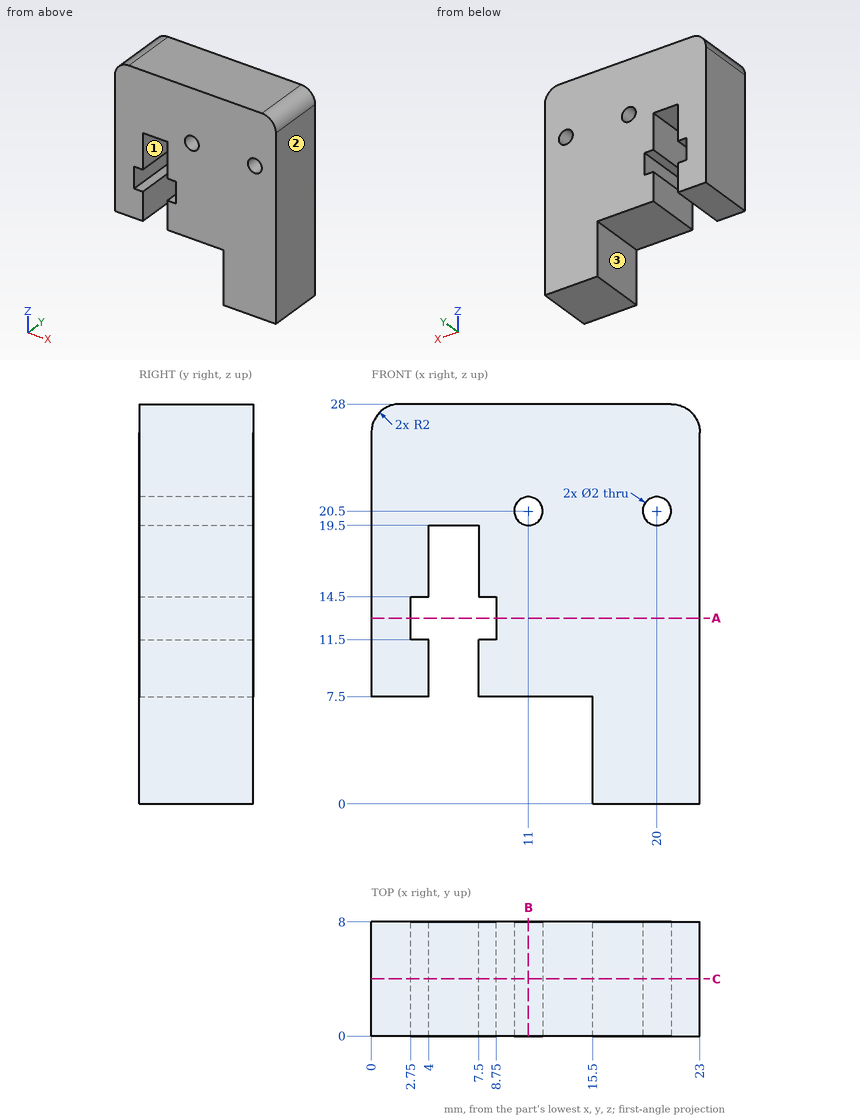
Job drawing, mm, ordinate dimensions from the low corner. One solid piece. A direction names the side the tool comes from. Round coordinates to 2 decimals unless told otherwise and drop trailing zeros. Loops run counter-clockwise (first coordinate to the right, second up) from the corner with the lowest first, then second, coordinate; pieces in that order, holes last. Notation, with made-up numbers: M 62.5,-34.75 L 113.5,-34.75 A26 ccw 113.5,-19.75 Z; hole C 89,5.25 d7. An arc over 180 degrees is marked long. One line per question, with ' | ' between items. Start each with the question number.
Item 1: Cut at A-A, the plane z = 13. Write the cut outline in (x, y), plus the area to 3 significant figures.
Item 2: Cut at C-C, the plane y = 4. Write the cut outline in (x, z).
Item 3: Wall check: line 1 (X direction, y = 4, z = 20.5); line 2 (X direction, y = 5, z = 10.75); line 3 (Z direction, x = 20, y = 4.5). Give the ranges that are in metal, low to high.
Item 4: Cut at B-B, the plane x = 11. Write the cut outline in (y, z).
Item 5: Pin check, flat tip, straight feed: pin 1 Ø0.6 at (x, y) = (3.5, 3.5) entering from -Z. Stop position of the tip, or through.
Item 6: Which spindle directions (+Z, -Z, +X, -X, +Y, -Y) get a long thin tool onto all of the face, cutting with end or side? Do the marked faces 1, 2 and 3. Say none if no direction does.
Responses:
1) outline: M 0,0 L 2.75,0 L 2.75,8 L 0,8 Z; M 8.75,0 L 23,0 L 23,8 L 8.75,8 Z | area: 136 mm²
2) outline: M 0,7.5 L 4,7.5 L 4,11.5 L 2.75,11.5 L 2.75,14.5 L 4,14.5 L 4,19.5 L 7.5,19.5 L 7.5,14.5 L 8.75,14.5 L 8.75,11.5 L 7.5,11.5 L 7.5,7.5 L 15.5,7.5 L 15.5,0 L 23,0 L 23,26 A2 ccw 21,28 L 2,28 A2 ccw 0,26 Z; hole C 11,20.5 d2; hole C 20,20.5 d2
3) line 1: x = 0 to 10, 12 to 19, 21 to 23 | line 2: x = 0 to 4, 7.5 to 23 | line 3: z = 0 to 19.5, 21.5 to 28
4) outline: M 0,7.5 L 8,7.5 L 8,19.5 L 0,19.5 Z; M 0,21.5 L 8,21.5 L 8,28 L 0,28 Z
5) pin 1: stops at z = 7.5
6) face 1: -Z, +Y, -Y | face 2: +Z, -Z, +X, +Y, -Y | face 3: -Z, -X, +Y, -Y
